CAD build for the part. Positions are in the model's coordinates, mm. A direction names the side the tool comes from. Give positions to 0.01 mm unless a question says otherwise; leave off trailing zeros. Loops run counter-clockwise (first coordinate to the right, second up) from the corner with the lowest first, then second, coordinate; pieces in that order, holes last.
Item 1: Saw through at D-D on z = 4. Give the cut face in (x, y).
Item 2: Drop flat-ended pins along their axis: P1, Ø8, axis at x = 58.5, y = 5, coming from the -Z side; P2, Ø8, axis at x = 37, y = 2, coming from the -Z side. Give the stop position or say it passes through.
Item 3: Mould opens along X. For faces 1 (the flat face through (32, 8, 1)), 2 (the flat face through (0, 0.2, 3.3)), 3 (the cylindrical face through (30.27, -11.29, 2.79)) say: released by +X, released by -X, zero draft, split by the parting line, or undercut.
Item 4: Saw through at C-C on y = -11. Give the cut face in (x, z).
Item 5: Probe probe 1 along Y at (x, z) = (58, 2.2); probe 2 along Y at (x, z) = (32.5, 4.3); probe 3 along Y at (x, z) = (18, 1.45). List the from-to ranges inside material, lowest first.
Item 6: Saw through at A-A on z = 0.95. Give the cut face in (x, y).
Item 7: Which spindle directions (+Z, -Z, +X, -X, +Y, -Y) get a long thin tool onto all of the face, cutting with end or side? Do faces 4 (the flat face through (32, -8, 1)), 5 (the cylindrical face through (5.48, -12.66, 2.79)). Say none if no direction does.
Item 8: Saw through at B-B on x = 58. Give the cut face in (y, z), plus the area to 3 significant figures.
Autodesk Inventor part; units mm, degrees
ref_plane "tbck_XY" through (0, 0, 0) normal (0, 0, 1) x (1, 0, 0)
ref_plane "tbck_YZ" through (0, 0, 0) normal (1, 0, 0) x (0, 1, 0)
ref_plane "tbck_ZX" through (0, 0, 0) normal (0, 1, 0) x (0, 0, 1)
sketch "Sketch_1" plane through (0, 0, 0) normal (0, 0, 1) x (1, 0, 0)
  line L0 (0, 16) -> (0, -16)
  line L1 (0, -16) -> (65, -16)
  line L2 (65, -16) -> (65, 16)
  line L3 (65, 16) -> (0, 16)
extrude "Extrusion1" add sketch "Sketch_1" along normal blind 5.5
sketch "Sketch2" plane through (0, 0, 0) normal (0, 0, -1) x (-1, 0, 0)
  point P0 (-7, 11)
hole "Hole1" at (7, 11, 0) direction (0, 0, 1) diameter 4.5 depth 5.5
pattern_linear "Rectangular Pattern1" count 3 spacing 25.5 along (1, 0, 0) count 2 spacing 22 along (0, -1, 0) of "Hole1"
sketch "Sketch_4" plane through (0, 0, 0) normal (1, 0, 0) x (0, 1, 0)
  line L0 (8, 2.9) -> (-8, 2.9)
  line L1 (-8, 2.9) -> (-8, 0)
  line L2 (-8, 0) -> (8, 0)
  line L3 (8, 0) -> (8, 2.9)
extrude "Extrusion2" cut sketch "Sketch_4" along normal blind 65
ref_plane "tbck_XY" through (0, 0, 0) normal (0, 0, 1) x (1, 0, 0)
ref_plane "tbck_YZ" through (0, 0, 0) normal (1, 0, 0) x (0, 1, 0)
ref_plane "tbck_ZX" through (0, 0, 0) normal (0, 1, 0) x (0, 0, 1)
ref_plane "tbck_hole_1_XY" through (7, -11, 5.5) normal (0, 0, 1) x (1, 0, 0)
ref_plane "tbck_hole_1_YZ" through (7, -11, 5.5) normal (1, 0, 0) x (0, 1, 0)
ref_plane "tbck_hole_1_ZX" through (7, -11, 5.5) normal (0, 1, 0) x (0, 0, 1)
ref_plane "tbck_hole_2_XY" through (32.5, -11, 5.5) normal (0, 0, 1) x (1, 0, 0)
ref_plane "tbck_hole_2_YZ" through (32.5, -11, 5.5) normal (1, 0, 0) x (0, 1, 0)
ref_plane "tbck_hole_2_ZX" through (32.5, -11, 5.5) normal (0, 1, 0) x (0, 0, 1)
ref_plane "tbck_hole_3_XY" through (58, -11, 5.5) normal (0, 0, 1) x (1, 0, 0)
ref_plane "tbck_hole_3_YZ" through (58, -11, 5.5) normal (1, 0, 0) x (0, 1, 0)
ref_plane "tbck_hole_3_ZX" through (58, -11, 5.5) normal (0, 1, 0) x (0, 0, 1)
ref_plane "tbck_holes_1_XY" through (7, 11, 5.5) normal (0, 0, 1) x (1, 0, 0)
ref_plane "tbck_holes_1_YZ" through (7, 11, 5.5) normal (1, 0, 0) x (0, 1, 0)
ref_plane "tbck_holes_1_ZX" through (7, 11, 5.5) normal (0, 1, 0) x (0, 0, 1)
ref_plane "tbck_holes_2_XY" through (32.5, 11, 5.5) normal (0, 0, 1) x (1, 0, 0)
ref_plane "tbck_holes_2_YZ" through (32.5, 11, 5.5) normal (1, 0, 0) x (0, 1, 0)
ref_plane "tbck_holes_2_ZX" through (32.5, 11, 5.5) normal (0, 1, 0) x (0, 0, 1)
ref_plane "tbck_holes_3_XY" through (58, 11, 5.5) normal (0, 0, 1) x (1, 0, 0)
ref_plane "tbck_holes_3_YZ" through (58, 11, 5.5) normal (1, 0, 0) x (0, 1, 0)
ref_plane "tbck_holes_3_ZX" through (58, 11, 5.5) normal (0, 1, 0) x (0, 0, 1)
properties part number "TBCKsupport_plate-MA5150_support_plate"
Results below:
1. outline: (0, -16) - (65, -16) - (65, 16) - (0, 16) - close; hole circle Ø4.5 at (7, -11); hole circle Ø4.5 at (7, 11); hole circle Ø4.5 at (32.5, -11); hole circle Ø4.5 at (32.5, 11); hole circle Ø4.5 at (58, -11); hole circle Ø4.5 at (58, 11)
2. P1: stops at z = 0
2. P2: stops at z = 2.9
3. face 1: zero draft
3. face 2: released by -X
3. face 3: undercut
4. outline: (0, 0) - (4.75, 0) - (4.75, 5.5) - (0, 5.5) - close; (9.25, 0) - (30.25, 0) - (30.25, 5.5) - (9.25, 5.5) - close; (34.75, 0) - (55.75, 0) - (55.75, 5.5) - (34.75, 5.5) - close; (60.25, 0) - (65, 0) - (65, 5.5) - (60.25, 5.5) - close
5. probe 1: y = -16 to -13.25, -8.75 to -8, 8 to 8.75, 13.25 to 16
5. probe 2: y = -16 to -13.25, -8.75 to 8.75, 13.25 to 16
5. probe 3: y = -16 to -8, 8 to 16
6. outline: (0, -16) - (65, -16) - (65, -8) - (0, -8) - close; (0, 8) - (65, 8) - (65, 16) - (0, 16) - close; hole circle Ø4.5 at (7, -11); hole circle Ø4.5 at (7, 11); hole circle Ø4.5 at (32.5, -11); hole circle Ø4.5 at (32.5, 11); hole circle Ø4.5 at (58, -11); hole circle Ø4.5 at (58, 11)
7. face 4: -Z, +X, -X
7. face 5: +Z, -Z
8. outline: (-16, 0) - (-13.25, 0) - (-13.25, 5.5) - (-16, 5.5) - close; (-8.75, 0) - (-8, 0) - (-8, 2.9) - (8, 2.9) - (8, 0) - (8.75, 0) - (8.75, 5.5) - (-8.75, 5.5) - close; (13.25, 0) - (16, 0) - (16, 5.5) - (13.25, 5.5) - close
8. area: 80.1 mm2
